from build123d import *

# Parameters (mm, degrees)
F1_DEPTH = 5
F2_R     = 4.99999


# Not quite as in the source:
# - a fillet or chamfer is up to 0.001 mm smaller than in the source, because OpenCascade refuses the exact size


with BuildPart() as f1:
    # F0 (on Top) → F1 (new body)
    with BuildSketch(Plane.XY):
        with BuildLine():
            Line((16.5, 0), (0, 0))
            Line((0, 0), (-16.5, 0))
            ThreePointArc((-16.5, 0), (-25.5, -9), (-34.5, 0))
            Line((-34.5, 0), (-55, 0))
            Line((-55, 0), (-55, -24))
            Line((-55, -24), (0, -24))
            Line((0, -24), (55, -24))
            Line((55, -24), (55, 0))
            Line((55, 0), (34.5, 0))
            ThreePointArc((34.5, 0), (25.5, -9), (16.5, 0))
        make_face()
    extrude(amount=F1_DEPTH)

    # F2 (radius 5 in the source; OpenCascade refuses exactly that, so slightly less here)
    f2_edges = [f1.edges().sort_by_distance(p)[0] for p in [
        (0, -24, 5),
        (-55, -12, 5),
        (55, -12, 5),
    ]]
    fillet(f2_edges, radius=F2_R)


solid = f1.part
Geometry: final body of the model. Coordinates: model frame, mm. Round coordinates to 2 decimals unless told otherwise and drop trailing zeros. Order: outer loops, then holes, each group sorted by start corner. A loop starts at its lowest first (then second) coordinate and runs counter-clockwise, first axis right, second up. Notation, with made-up numbers: (87, 61) -> (91, 61) arc R29 ccw to (91, 99) -> close; hole circle Ø3 at (84.25, -11.5). An arc over 180 degrees is marked (long way). Put each result on its own line as item: value. Start each with the question number.
Q1. First-contact query: pin 1 (3 mm diameter, centred on y = -5, z = 4, fed in from -X). Flat tip, straight axial feed; report the tip coordinate or a pass-through.
Q2. Line query: probe 1 along X at (y, z) = (-1.5, 3.7); probe 2 along X at (y, z) = (-3.25, 2.3); probe 3 along Y at (x, z) = (39.5, 3). Output: solid intervals per line, ascending.
Q3. Section A-A on z = 3. Return the cut outline in (x, y), and give its area (3 significant figures).
Q4. Section C-C on y = -5.5. Give the number of separate pieces and of enclosed holes in the cut face, and give its area (3 significant figures).
Q5. Pull-direction query (X, two-part tool) for faces 1 (the flat face through (-1, -9, 5)), 2 (the cylindrical face through (25.698, -8.998, 2.465)), 3 (the cylindrical face through (-54, -12, 3)); classes: +X half, -X half, draft (parallel to the pull), parting line (faces both ways), or undercut.
Ans:
1. pin 1: stops at x = -54.33
2. probe 1: x = -53.36 to -34.37, -16.63 to 16.63, 34.37 to 53.36
2. probe 2: x = -54.44 to -33.89, -17.11 to 17.11, 33.89 to 54.44
2. probe 3: y = -23 to 0
3. outline: (-54, -23) -> (54, -23) -> (54, 0) -> (34.5, 0) arc R9 cw to (16.5, 0) -> (-16.5, 0) arc R9 cw to (-34.5, 0) -> (-54, 0) -> close
3. area: 2,230 mm2
4. separate pieces: 3
4. enclosed holes: 0
4. area: 397 mm2
5. face 1: draft
5. face 2: undercut
5. face 3: -X half
